Read the model definition and answer for the solid it produces. Units are mm, in the model's axes. Coordinates: 2 decimals unless noted, no trailing zeros. Write each loop counter-clockwise with the first axis right and the second up, starting at its lowest first coordinate (ties: lowest second). Pieces come first, ordered by that corner, then holes.
Item 1: Section B-B (x = -9) is taken. Give the vertices of the cut face in (y, z).
Item 2: Determine the mould class of faces 1 (the face through (60.42, -10.06, 0.89)), 2 (the face through (-25.568, -9.594, 0.887)), 3 (the face through (1, -3, 0)) for opening direction X: released by +X, released by -X, zero draft, split by the parting line, or undercut.
Item 3: Section C-C (z = 0.35) is taken. State how many separate pieces and enclosed holes the cut face has, then the cut area to 3 significant figures.
Item 4: Section D-D (x = -27) is taken. Give the vertices of the cut face in (y, z), then the cut area to 3 significant figures.
Item 5: Straight lines are drawn through the part: probe 1 along X at (y, z) = (-13.5, 1.5); probe 2 along X at (y, z) = (-14.5, 0.15); probe 3 along Y at (x, z) = (-9, 0.75). For each, find the intervals that lie inside material, in ascending order.
Item 6: Section A-A (y = -9) is taken. Give the vertices of the cut face in (x, z), then the cut area to 3 significant figures.
Item 7: Each of these flat-tipped pins is pushed along its axis until it touches: P1, Ø2.5, axis at x = 53.5, y = -9, coming from the -Z side; P2, Ø0.5, axis at x = -38, z = 0.5, coming from the -Y side; P3, Ø1, axis at x = -21, z = 1, coming from the +Y side. Where does it stop, or does it pass through?
from build123d import *

# Parameters (mm, degrees)
SKETCH_1_R      = 1.55
EXTRUDE_1_DEPTH = 1.8
FILLET_1_R      = 2


with BuildPart() as part:
    # 草图1 → 凸台-拉伸1 (new body)
    with BuildSketch(Plane.XY):
        with BuildLine():
            Line((-19, 10.5), (19, 10.5))
            ThreePointArc((19, 10.5), (19.856766341, 10.426048258), (20.688188937, 10.206380575))
            Line((20.688188937, 10.206380575), (55.863464512, -2.411067196))
            ThreePointArc((55.863464512, -2.411067196), (60.396467561, -10.199472878), (53.5, -16))
            Line((53.5, -16), (42.25, -16))
            Line((42.25, -16), (40.57664504, -10))
            Line((40.57664504, -10), (35.42335496, -10))
            Line((35.42335496, -10), (33.75, -16))
            Line((33.75, -16), (-33.75, -16))
            Line((-33.75, -16), (-35.42335496, -10))
            Line((-35.42335496, -10), (-40.57664504, -10))
            Line((-40.57664504, -10), (-42.25, -16))
            Line((-42.25, -16), (-53.5, -16))
            ThreePointArc((-53.5, -16), (-60.396467561, -10.199472878), (-55.863464512, -2.411067196))
            Line((-55.863464512, -2.411067196), (-20.688188937, 10.206380575))
            ThreePointArc((-20.688188937, 10.206380575), (-19.856766341, 10.426048258), (-19, 10.5))
        make_face()
        with Locations((-27, -9)):
            Circle(SKETCH_1_R, mode=Mode.SUBTRACT)
        with Locations((-9, -9)):
            Circle(SKETCH_1_R, mode=Mode.SUBTRACT)
        with Locations((13, -9)):
            Circle(SKETCH_1_R, mode=Mode.SUBTRACT)
        with Locations((30, -9)):
            Circle(SKETCH_1_R, mode=Mode.SUBTRACT)
        with Locations((0, 7)):
            Circle(SKETCH_1_R, mode=Mode.SUBTRACT)
        with Locations((-53.5, -9)):
            Circle(SKETCH_1_R, mode=Mode.SUBTRACT)
        with Locations((53.5, -9)):
            Circle(SKETCH_1_R, mode=Mode.SUBTRACT)
        with Locations((-19, 5.5)):
            Circle(SKETCH_1_R, mode=Mode.SUBTRACT)
        with Locations((19, 5.5)):
            Circle(SKETCH_1_R, mode=Mode.SUBTRACT)
    extrude(amount=EXTRUDE_1_DEPTH)

    # 圆角1
    fillet_1_edges = [part.edges().sort_by_distance(p)[0] for p in [
        (42.25, -16, 0.9),
        (40.57664504, -10, 0.9),
        (35.42335496, -10, 0.9),
        (33.75, -16, 0.9),
        (-33.75, -16, 0.9),
        (-35.42335496, -10, 0.9),
        (-40.57664504, -10, 0.9),
        (-42.25, -16, 0.9),
    ]]
    fillet(fillet_1_edges, radius=FILLET_1_R)


solid = part.part
Established:
1. outline: (-16, 0) - (-10.55, 0) - (-10.55, 1.8) - (-16, 1.8) - close; (-7.45, 0) - (10.5, 0) - (10.5, 1.8) - (-7.45, 1.8) - close
2. face 1: released by +X
2. face 2: undercut
2. face 3: zero draft
3. separate pieces: 1
3. enclosed holes: 9
3. area: 2,430 mm2
4. outline: (-16, 0) - (-10.55, 0) - (-10.55, 1.8) - (-16, 1.8) - close; (-7.45, 0) - (7.94, 0) - (7.94, 1.8) - (-7.45, 1.8) - close
4. area: 37.5 mm2
5. probe 1: x = -58.86 to -41.55, -34.45 to 34.45, 41.55 to 58.86
5. probe 2: x = -57.83 to -41.83, -34.17 to 34.17, 41.83 to 57.83
5. probe 3: y = -16 to -10.55, -7.45 to 10.5
6. outline: (-60.5, 0) - (-55.05, 0) - (-55.05, 1.8) - (-60.5, 1.8) - close; (-51.95, 0) - (-28.55, 0) - (-28.55, 1.8) - (-51.95, 1.8) - close; (-25.45, 0) - (-10.55, 0) - (-10.55, 1.8) - (-25.45, 1.8) - close; (-7.45, 0) - (11.45, 0) - (11.45, 1.8) - (-7.45, 1.8) - close; (14.55, 0) - (28.45, 0) - (28.45, 1.8) - (14.55, 1.8) - close; (31.55, 0) - (51.95, 0) - (51.95, 1.8) - (31.55, 1.8) - close; (55.05, 0) - (60.5, 0) - (60.5, 1.8) - (55.05, 1.8) - close
6. area: 184 mm2
7. P1: passes through
7. P2: stops at y = -10
7. P3: stops at y = 10.27
